The drawing under review shows one solid part. Ordinate dimensions are in mm from its lowest x, y, z. A direction names the side the tool comes from. Coordinates: 2 decimals unless noted, no trailing zeros. Order: outer loops, then holes, each group sorted by start corner. A loop starts at its lowest first (then second) coordinate and runs counter-clockwise, first axis right, second up. Notation, with made-up numbers: (74, 24) -> (113, 24) arc R27 ccw to (113, 41) -> close; hole circle Ø9 at (35, -2). An arc over 180 degrees is marked (long way). Use a Markdown table: item, result. Add a question column.
Q1. Add section A-A (y = 177.8). State the section outline as (x, z) points.
Q2. Wall thickness on probe 1 along Y at (x, z) = (26, 1.5); probe 2 along Y at (x, z) = (34, 8.25); probe 3 along Z at (x, y) = (27, 274): over which ranges is each line inside the solid? List them lowest first.
Q3. Add section C-C (x = 25.4). State the section outline as (y, z) points, then the cut area to 3 significant figures.
Q4. Add section D-D (x = 7). State the section outline as (y, z) points.
Q5. Machinability: for the marked faces 1 and 2, which of the approach directions +Z, -Z, +X, -X, +Y, -Y give a long, thin tool a straight path to every point of the face, cutting with its end or side? Answer none if there is none.
Q6. Add section B-B (z = 10.25). State the section outline as (x, y) points.
Q7. Insertion check: pin 1 (3 mm diameter, centred on x = 42, y = 215, fed in from +Z); pin 2 (7 mm diameter, centred on x = 32.5, z = 9.5, fed in from -Y). Each pin has a flat end and moves straight along its axis. Give the tip position at first contact, or say it passes through.
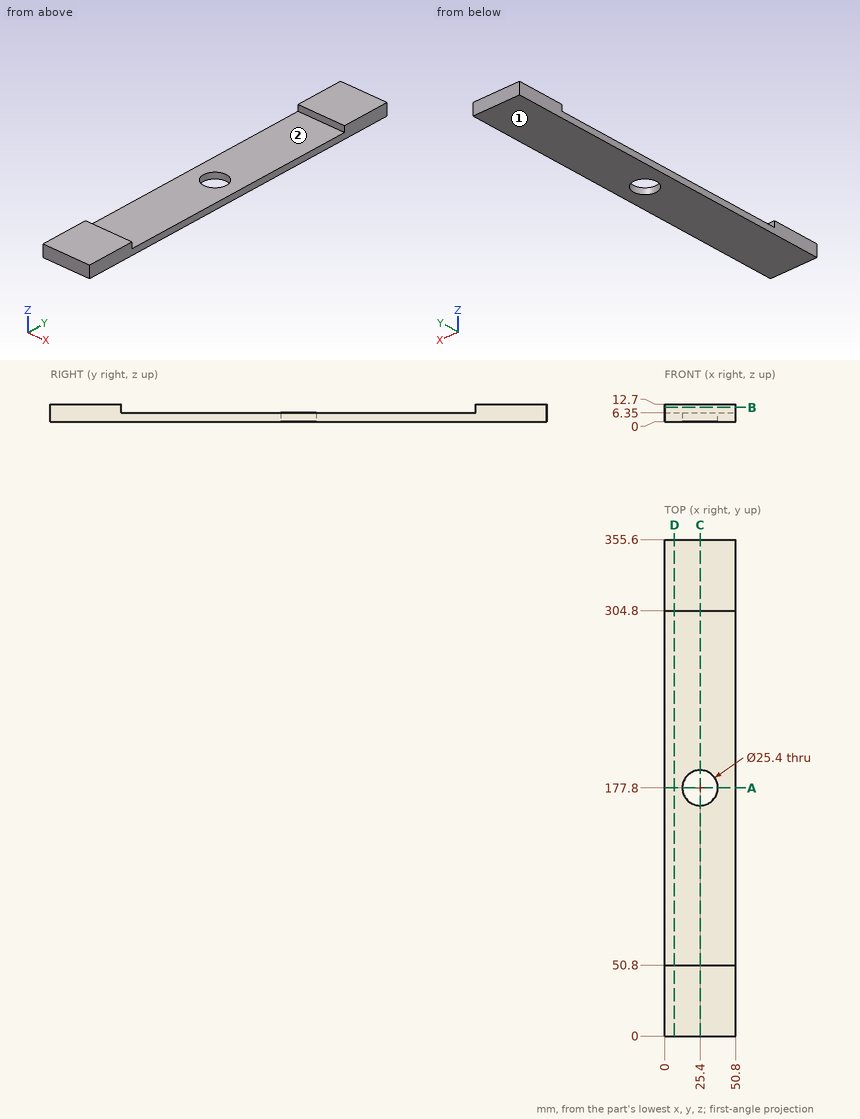
Established:
| question | item | result |
|---|---|---|
| 1 | outline | (0, 0) -> (12.7, 0) -> (12.7, 6.35) -> (0, 6.35) -> close; (38.1, 0) -> (50.8, 0) -> (50.8, 6.35) -> (38.1, 6.35) -> close |
| 2 | probe 1 | 0 to 165.11, 190.49 to 355.6 |
| 2 | probe 2 | 0 to 50.8, 304.8 to 355.6 |
| 2 | probe 3 | 0 to 6.35 |
| 3 | outline | (0, 0) -> (165.1, 0) -> (165.1, 6.35) -> (50.8, 6.35) -> (50.8, 12.7) -> (0, 12.7) -> close; (190.5, 0) -> (355.6, 0) -> (355.6, 12.7) -> (304.8, 12.7) -> (304.8, 6.35) -> (190.5, 6.35) -> close |
| 3 | area | 2,740 mm^2 |
| 4 | outline | (0, 0) -> (355.6, 0) -> (355.6, 12.7) -> (304.8, 12.7) -> (304.8, 6.35) -> (50.8, 6.35) -> (50.8, 12.7) -> (0, 12.7) -> close |
| 5 | face 1 | -Z, +X, -X, +Y, -Y |
| 5 | face 2 | +Z, +X, -X |
| 6 | outline | (0, 0) -> (50.8, 0) -> (50.8, 50.8) -> (0, 50.8) -> close; (0, 304.8) -> (50.8, 304.8) -> (50.8, 355.6) -> (0, 355.6) -> close |
| 7 | pin 1 | z = 6.35 |
| 7 | pin 2 | y = 0 |
